Autodesk Inventor part; units mm, degrees
ref_plane "YZ Plane" through (0, 0, 0) normal (1, 0, 0) x (0, 1, 0)
ref_plane "XZ Plane" through (0, 0, 0) normal (0, 1, 0) x (-1, 0, 0)
ref_plane "XY Plane" through (0, 0, 0) normal (0, 0, 1) x (1, 0, 0)
sketch "Sketch2" plane through (0, 0, 0) normal (0, 0, 1) x (1, 0, 0)
  line L0 (0, 0) -> (0, 8.3073) construction
  line L1 (2, 0) -> (2, 7.5)
  line L2 (2, 7.5) -> (4.1473, 7.5)
  line L3 (4.1473, 7.5) -> (4.5, 5.5)
  line L4 (4.5, 5.5) -> (4.5, 4)
  line L5 (4.5, 4) -> (4, 4)
  line L6 (4, 4) -> (4, 0)
  line L7 (4, 0) -> (2, 0)
  dimension "d1" = 4
  dimension "d2" = 7.5
  dimension "d3" = 3.5
  dimension "d4" = 10
  dimension "d5" = 8
  dimension "d6" = 9
  dimension "d7" = 2
revolve "Revolution1" add sketch "Sketch2" angle 360 about axis through (0, 0, 0) along (0, 1, 0)
sketch "Sketch3" plane through (0, 0, 0) normal (0, 0, 1) x (1, 0, 0)
  line L0 (0, 0) -> (0, 7.5)
  line L1 (-4.1473, 7.5) -> (4.1473, 7.5)
  circle A0 centre (-8, 5) radius 1.25
  circle A1 centre (-8, 5) radius 2.5
  line L2 (-4.5, 4) -> (4.5, 4)
  line L3 (-7.25, 4) -> (-4.5, 4)
  line L4 (-4.5, 5.5) -> (-4.5, 4)
  line L5 (-4.5, 5.5) -> (-5.5505, 5.5)
  circle A2 centre (8, 5) radius 1.25
  circle A3 centre (8, 5) radius 2.5
  line L6 (7.25, 4) -> (4.5, 4)
  line L7 (4.5, 5.5) -> (5.5505, 5.5)
  line L8 (-10.2913, 4) -> (-9.1121, 4.4292)
  line L9 (-8, 5) -> (-8, -2.6119) construction
  line L10 (-4.5, 5.5) -> (-2.8248, 5.5)
  line L11 (-4.5, 5.5) -> (4.5, 5.5)
  line L12 (-2.8248, 4) -> (-2.8248, 5.5)
  line L13 (4.5, 5.5) -> (2.7431, 5.5)
  line L14 (2.7431, 5.5) -> (2.7431, 4)
  line L15 (10.2913, 4) -> (9.1121, 4.4292)
  line L16 (-6.75, 5) -> (-6.75, 4)
  line L17 (6.75, 5) -> (6.75, 4)
  dimension "d9" = 5
  dimension "d10" = 2.5
  dimension "d11" = 16
  dimension "d12" = 70
extrude "Extrusion1" add sketch "Sketch3" along normal mid plane 13 contours L2 L4 L10 L12 | L14 L11 L7 A3 L6 L2 | L3 A1 L5 L4 | L3 L16 A0 L8 A1 | A3 L15 A2 L17 L6
sketch "Sketch4" plane through (2.7431, 4, -6.5) normal (0, -1, 0) x (1, 0, 0)
  line L0 (-9.4931, 0) -> (-9.4931, 13)
  line L1 (4.0069, 13) -> (4.0069, 0)
  line L2 (5.2569, -3.5) -> (-10.7431, -3.5)
  line L3 (-2.7431, -3.5) -> (-2.7431, 6.5)
  line L4 (5.2569, -3.5) -> (5.2569, 0)
  line L5 (0, 0) -> (2.8074, 0)
  line L6 (5.2569, 0) -> (0, 0)
  line L7 (0, 0) -> (0, 2.8945)
  arc A0 (-5.5678, 2.997) -> (0, 2.9327) centre (-2.7431, 6.5) ccw
  line L8 (-10.7431, -3.5) -> (-10.7431, 0)
  line L9 (-8.2936, 0) -> (-5.5678, 0)
  line L10 (-10.7431, 0) -> (-5.5678, 0)
  line L11 (-5.5678, 0) -> (-5.5678, 2.997)
  line L12 (-5.5678, 0) -> (-5.5678, 2.997)
  line L13 (-2.7431, 6.5) -> (4.0069, 6.5)
  line L14 (5.2569, 16.5) -> (-10.7431, 16.5)
  line L15 (5.2569, 16.5) -> (5.2569, 13)
  line L16 (0, 13) -> (2.8074, 13)
  line L17 (5.2569, 13) -> (0, 13)
  line L18 (0, 13) -> (0, 10.1055)
  arc A1 (0, 10.0673) -> (-5.5678, 10.003) centre (-2.7431, 6.5) ccw
  line L19 (-10.7431, 16.5) -> (-10.7431, 13)
  line L20 (-8.2936, 13) -> (-5.5678, 13)
  line L21 (-10.7431, 13) -> (-5.5678, 13)
  line L22 (-5.5678, 13) -> (-5.5678, 10.003)
  line L23 (-5.5678, 13) -> (-5.5678, 10.003)
  arc A2 (0, 2.9327) -> (0, 10.0673) centre (-2.7431, 6.5) ccw
  arc A3 (-5.5678, 10.003) -> (-5.5678, 2.997) centre (-2.7431, 6.5) ccw
  point P0 (-2.7431, 16.5)
  dimension "d15" = 16
  dimension "d21" = 20
extrude "Extrusion2" add sketch "Sketch4" against normal up to surface (1.5 mm away) contours L10 L9 L11 A0 L3 L2 L8 | L21 L19 L14 L15 L17 L1 L13 A2 A1 L22 L20 | L3 A0 A2 L13 L1 L6 L4 L2
sketch "Sketch5" plane through (5.5505, 5.5, 6.5) normal (0, 1, 0) x (1, 0, 0)
  line L0 (-5.5505, 6.5) -> (4.9752, 6.5)
  line L1 (-13.5505, 16.5) -> (2.4495, 16.5)
  line L2 (2.4495, 16.5) -> (-13.5505, 16.5)
  line L3 (-13.5505, 16.5) -> (-13.5505, 14.5)
  line L4 (-13.5505, 14.5) -> (2.4495, 14.5)
  line L5 (2.4495, 14.5) -> (2.4495, 16.5)
  line L6 (-13.5505, -3.5) -> (2.4495, -3.5)
  line L7 (2.4495, -3.5) -> (-13.5505, -3.5)
  line L8 (-13.5505, -3.5) -> (-13.5505, -1.5)
  line L9 (-13.5505, -1.5) -> (2.4495, -1.5)
  line L10 (2.4495, -1.5) -> (2.4495, -3.5)
  dimension "d18" = 16
extrude "Extrusion3" add sketch "Sketch5" along normal up to surface (2 mm away)
properties part number "18102021-002-06" material "Stainless Steel"
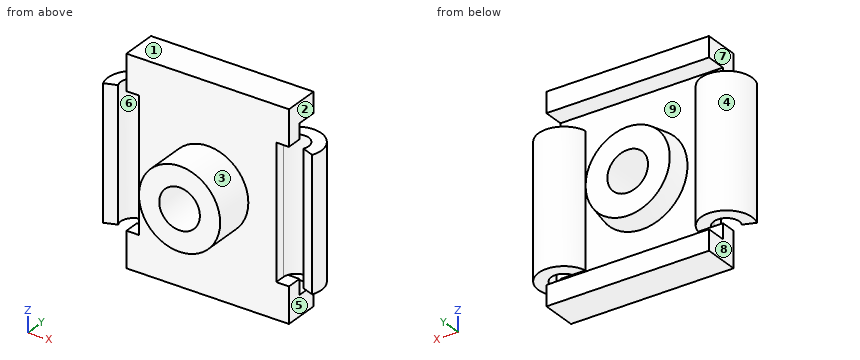
Read the model definition and answer for the solid it produces. Units are mm, in the model's axes. Face numbers are marked on the shaded views. A direction names the side the tool comes from. Give positions to 0.01 mm unless a question says otherwise; leave off trailing zeros. Write each loop counter-clockwise with the first axis right and the second up, starting at its lowest first coordinate (ties: lowest second). Pieces come first, ordered by that corner, then holes. Notation, with made-up numbers: (-26, 1.25) - (28, 1.25) arc R19 ccw to (28, 16.25) - close; hole circle Ø8 at (88.5, 29). An arc over 180 degrees is marked (long way). Return JSON: item names as keys, results as strings.
Q1. A cutting plane is placed at D-D, the plane x = -8.5. Determine the outline of the cut face in (y, z).
Reply:
{"outline": "(6.15, -6.5) - (7.45, -6.5) - (7.45, 6.5) - (6.15, 6.5) - close"}
Q2. Given P1, Ø1.5, axis at x = 7, z = -1, coming from the -Y side; P2, Ø1, axis at y = 3, z = -3, coming from the +X side; P3, Ø2, axis at y = 1, z = 0, coming from the -X side, each flat-ended and moving along its own axis, determine where each tip first touches the part or whether it passes through.
Reply:
{"P1": "y = 4", "P2": "x = 3.12", "P3": "x = -4"}
Q3. For a pull along Z with two mould halves and no side action, classify the marked faces 1, 2, 3 and 4 as released by +Z, released by -Z, zero draft, split by the parting line, or undercut.
Reply:
{"face 1": "released by +Z", "face 2": "zero draft", "face 3": "split by the parting line", "face 4": "undercut"}
Q4. For the marked faces 5, 6, 7, 8 and 9, determine the directions among +Z, -Z, +X, -X, +Y, -Y from which every point of the face is accessible in a straight line to the end or side of a thin tool.
Reply:
{"face 5": "-Z, +X, +Y, -Y", "face 6": "none", "face 7": "+Z, -X, +Y, -Y", "face 8": "-Z, -X, +Y, -Y", "face 9": "+Y"}
Q5. A cutting plane is placed at C-C, the plane z = -6.25. Determine the outline of the cut face in (x, y).
Reply:
{"outline": "(-10.29, 4) - (-9.11, 4.43) arc R1.25 cw (long way) to (-6.75, 5) - (-6.75, 4) - (6.75, 4) - (6.75, 5) arc R1.25 cw (long way) to (9.11, 4.43) - (10.29, 4) arc R2.5 ccw (long way) to (5.55, 5.5) - (-5.55, 5.5) arc R2.5 ccw (long way) to start"}
Q6. A cutting plane is placed at B-B, the plane z = 0. Determine the outline of the cut face in (x, y).
Reply:
{"outline": "(-10.29, 4) - (-9.11, 4.43) arc R1.25 cw (long way) to (-6.75, 5) - (-6.75, 4) - (-4, 4) - (-4, 0) - (-2, 0) - (-2, 7.5) - (-4.15, 7.5) - (-4.5, 5.5) - (-5.55, 5.5) arc R2.5 ccw (long way) to start; (2, 0) - (4, 0) - (4, 4) - (6.75, 4) - (6.75, 5) arc R1.25 cw (long way) to (9.11, 4.43) - (10.29, 4) arc R2.5 ccw (long way) to (5.55, 5.5) - (4.5, 5.5) - (4.15, 7.5) - (2, 7.5) - close"}
Q7. Consider line 1 along Z through (x, y) = (-4.5, 6.25); line 2 along X through (y, z) = (2.5, 0); line 3 along X through (y, z) = (5.25, 0). Determine where each line is inside the solid, lowest interval first. Write a range as [from, to].
Reply:
{"line 1": "[-10, -8], [8, 10]", "line 2": "[-4, -2], [2, 4]", "line 3": "[-10.49, -9.22], [-6.78, -2], [2, 6.78], [9.22, 10.49]"}
Q8. A cutting plane is placed at A-A, the plane y = 1.5. Determine the outline of the cut face in (x, z), and give its area (3 significant figures).
Reply:
{"outline": "circle Ø8 at (0, 0); hole circle Ø4 at (0, 0)", "area": "37.7 mm²"}
